from build123d import *

# Parameters (mm, degrees)
F0_R     = 25.4
F0_R_2   = 22.225
F2_DEPTH = 25.4
F3_D     = 3.175


with BuildPart() as f2:
    # F0 (on Front) → F2 (new body)
    with BuildSketch(Plane.XZ):
        Circle(F0_R)
        Circle(F0_R_2, mode=Mode.SUBTRACT)
        Circle(F0_R_2)
    extrude(amount=F2_DEPTH)

    # F3 (through all)
    with Locations(Plane(origin=(0, 0, 0), x_dir=(1, 0, 0), z_dir=(0, 1, 0))):
        with Locations((0, 17.526003), (16.001999, 0), (0, -17.525999), (-17.335502, 0)):
            Hole(F3_D / 2)


solid = f2.part
The listing builds one solid part. Answer for the finished solid, in the listing's coordinates (mm). Round coordinates to 2 decimals unless told otherwise and drop trailing zeros. Order: outer loops, then holes, each group sorted by start corner. A loop starts at its lowest first (then second) coordinate and runs counter-clockwise, first axis right, second up. Notation, with made-up numbers: (57, -6.5) -> (84, -6.5) arc R16 ccw to (84, 13.5) -> close; hole circle Ø4 at (-4.75, -17.5). An arc over 180 degrees is marked (long way). Write each question's results on one line, items separated by ' | '. Start each with the question number.
Q1. The mould has two halves that part along X. Classify faces 1 (the cylindrical face through (-18.85, -12.88, -0.48)), 2 (the flat face through (0, 0, 0)), 3 (the cylindrical face through (-5.506, -12.522, -24.796)), 4 (the cylindrical face through (1.26, -12.88, -16.56)): pulls with the +X half, pulls with the -X half, needs draft (parallel to the pull), parting line crosses it, or undercut.
Q2. Each of these flat-tipped pins is pushed along its axis until it touches: pin 1 (8 mm diameter, centred on x = -10, y = -7.5, fed in from -Z); pin 2 (12 mm diameter, centred on y = -9.5, z = -13.5, fed in from +X); pin 3 (2 mm diameter, centred on x = -12, y = -9.5, fed in from +Z); pin 4 (1.9 mm diameter, centred on x = 0, z = 17.53, fed in from -Y). Where does it stop, or does it pass through?
Q3. Find section C-C (y = -3.5). Determine the outline of the cut face in (x, z) (1 decimal), then the cut area to 3 significant figures.
Q4. Find section B-B (x = 0). Determine the outline of the cut face in (y, z), then the cut area to 3 significant figures.
Q5. Find section A-A (z = 0). Determine the outline of the cut face in (x, y), then the cut area to 3 significant figures.
Q6. Find section D-D (x = -11). Determine the outline of the cut face in (y, z).
Q7. Straight lines are drawn through the part: probe 1 along Z at (x, y) = (0, -10); probe 2 along X at (y, z) = (-7.75, -0.5); probe 3 along X at (y, z) = (-6.25, -17.5). For each, find the intervals that lie inside material, in ascending order. Write a range as from..to.
Worked answers:
1) face 1: undercut | face 2: needs draft | face 3: parting line crosses it | face 4: undercut
2) pin 1: stops at z = -24.68 | pin 2: stops at x = 24.27 | pin 3: stops at z = 22.89 | pin 4: passes through
3) outline: circle Ø50.8 at (0, 0); hole circle Ø3.2 at (-17.3, 0); hole circle Ø3.2 at (0, -17.5); hole circle Ø3.2 at (0, 17.5); hole circle Ø3.2 at (16, 0) | area: 2,000 mm2
4) outline: (-25.4, -25.4) -> (0, -25.4) -> (0, -19.11) -> (-25.4, -19.11) -> close; (-25.4, -15.94) -> (0, -15.94) -> (0, 15.94) -> (-25.4, 15.94) -> close; (-25.4, 19.11) -> (0, 19.11) -> (0, 25.4) -> (-25.4, 25.4) -> close | area: 1,130 mm2
5) outline: (-25.4, -25.4) -> (-18.92, -25.4) -> (-18.92, 0) -> (-25.4, 0) -> close; (-15.75, -25.4) -> (14.41, -25.4) -> (14.41, 0) -> (-15.75, 0) -> close; (17.59, -25.4) -> (25.4, -25.4) -> (25.4, 0) -> (17.59, 0) -> close | area: 1,130 mm2
6) outline: (-25.4, -22.89) -> (0, -22.89) -> (0, 22.89) -> (-25.4, 22.89) -> close
7) probe 1: z = -25.4..-19.11, -15.94..15.94, 19.11..25.4 | probe 2: x = -25.4..-18.84, -15.83..14.5, 17.51..25.4 | probe 3: x = -18.41..-1.59, 1.59..18.41
